```python
from build123d import *

# Parameters (mm, degrees)
SKETCH1_W           = 35
SKETCH1_H           = 22.25
BOSS_EXTRUDE1_DEPTH = 11.5
SKETCH2_R           = 2.2
CUT_EXTRUDE1_DEPTH  = 31.554255023
LPATTERN1_COUNT     = 3
LPATTERN1_PITCH     = 12.7
SKETCH3_W           = 20
SKETCH3_H           = 22.25
BOSS_EXTRUDE2_DEPTH = 50
SKETCH4_W           = 16.4
SKETCH4_H           = 20
BOSS_EXTRUDE3_DEPTH = 44.87
CHAMFER1_SIZE       = 20
SKETCH5_W           = 20
SKETCH5_H           = 22.25
BOSS_EXTRUDE4_DEPTH = 15
CHAMFER2_SIZE       = 12
SKETCH6_W           = 16.4
SKETCH6_H           = 24
BOSS_EXTRUDE5_DEPTH = 18
BOSS_EXTRUDE6_DEPTH = 16.4
SKETCH11_R          = 2.35
CUT_EXTRUDE4_DEPTH  = 119.961327802
SKETCH12_R          = 4.2
CUT_EXTRUDE5_DEPTH  = 16


with BuildPart() as part:
    # Sketch1 → Boss-Extrude1 (new body)
    with BuildSketch(Plane(origin=(0, 0, 0), x_dir=(0, 0, -1), z_dir=(1, 0, 0))):
        Rectangle(SKETCH1_W, SKETCH1_H)
    extrude(amount=BOSS_EXTRUDE1_DEPTH)

    # Sketch2 → Cut-Extrude1 (cut, through all)
    with BuildSketch(Plane(origin=(0, 11.125, 0), x_dir=(1, 0, 0), z_dir=(0, 1, 0))):
        with Locations(Location((5.15, -10.5, 0), (0, 0, 270))):
            Circle(SKETCH2_R)
    cut_extrude1 = extrude(amount=-CUT_EXTRUDE1_DEPTH, mode=Mode.SUBTRACT)

    # LPattern1: Cut-Extrude1 ×3
    with Locations(*[(0, 0, -i * LPATTERN1_PITCH) for i in range(1, LPATTERN1_COUNT)]):
        add(cut_extrude1, mode=Mode.SUBTRACT)


with BuildPart() as body_2:
    # Mirror3: mirrored copy
    add(part.part.mirror(Plane(origin=(43.25, 0, 0), x_dir=(0, 0, 1), z_dir=(1, 0, 0))))


with BuildPart() as part_1:
    add(part.part)

    # Sketch3 → Boss-Extrude2 (add)
    with BuildSketch(Plane(origin=(11.5, 0, 0), x_dir=(0, 0, -1), z_dir=(1, 0, 0))):
        with Locations((7.5, 0)):
            Rectangle(SKETCH3_W, SKETCH3_H)
    extrude(amount=BOSS_EXTRUDE2_DEPTH)

    # Sketch4 → Boss-Extrude3 (add)
    with BuildSketch(Plane(origin=(0, 11.125, 0), x_dir=(1, 0, 0), z_dir=(0, 1, 0))):
        with Locations((53.3, 7.5)):
            Rectangle(SKETCH4_W, SKETCH4_H)
    extrude(amount=BOSS_EXTRUDE3_DEPTH)

    # Chamfer1
    chamfer1_edges = [part_1.edges().sort_by_distance(p)[0] for p in [
        (45.1, 11.125, -7.5),
    ]]
    chamfer(chamfer1_edges, length=CHAMFER1_SIZE)

    add(body_2.part)  # Boss-Extrude4 merges body 2
    # Sketch5 → Boss-Extrude4 (add)
    with BuildSketch(Plane(origin=(61.5, 0, 0), x_dir=(0, 0, -1), z_dir=(1, 0, 0))):
        with Locations((7.5, 0)):
            Rectangle(SKETCH5_W, SKETCH5_H)
    extrude(amount=BOSS_EXTRUDE4_DEPTH)

    # Chamfer2
    chamfer2_edges = [part_1.edges().sort_by_distance(p)[0] for p in [
        (61.5, 11.125, -7.5),
    ]]
    chamfer(chamfer2_edges, length=CHAMFER2_SIZE)

    # Sketch6 → Boss-Extrude5 (add)
    with BuildSketch(Plane(origin=(0, 0, -17.5), x_dir=(-1, 0, 0), z_dir=(0, 0, -1))):
        with Locations((-53.3, 43.995)):
            Rectangle(SKETCH6_W, SKETCH6_H)
    extrude(amount=BOSS_EXTRUDE5_DEPTH)

    # Sketch7 → Boss-Extrude6 (add)
    with BuildSketch(Plane(origin=(61.5, 0, 0), x_dir=(0, 0, -1), z_dir=(1, 0, 0))):
        Polygon((35.5, 31.995), (59.5, 55.995), (35.5, 55.995), align=None)
    extrude(amount=-BOSS_EXTRUDE6_DEPTH)

    # Sketch11 → Cut-Extrude4 (cut, through all)
    with BuildSketch(Plane(origin=(0, -1.7525, -1.7525), x_dir=(1, 0, 0), z_dir=(0, -0.7071067811865509, -0.7071067811865441))):
        with Locations(Location((52.778087488, -58.643931452, 0), (0, 0, 270))):
            Circle(SKETCH11_R)
    extrude(amount=-CUT_EXTRUDE4_DEPTH, mode=Mode.SUBTRACT)

    # Sketch12 → Cut-Extrude5 (cut)
    with BuildSketch(Plane(origin=(0, 17.449710754, 17.449710754), x_dir=(1, 0, 0), z_dir=(0, 0.7071067811865464, 0.7071067811865488))):
        with Locations(Location((52.778087488, 58.643931452, 0), (0, 0, 270))):
            Circle(SKETCH12_R)
    extrude(amount=-CUT_EXTRUDE5_DEPTH, mode=Mode.SUBTRACT)


solid = part_1.part
```
The listing builds one solid part. Answer for the finished solid, in the listing's coordinates (mm). A direction names the side the tool comes from. Give positions to 0.01 mm unless a question says otherwise; leave off trailing zeros. Order: outer loops, then holes, each group sorted by start corner. A loop starts at its lowest first (then second) coordinate and runs counter-clockwise, first axis right, second up. Notation, with made-up numbers: (-35, 22) - (12, 22) arc R19 cw to (12, 43) - close; hole circle Ø11 at (70.25, 73.5). An arc over 180 degrees is marked (long way). Use one line per item in the form item = value. Start each with the question number.
(1) Flat-ended cylindrical pins translate along their axes: pin 1 Ø7.5 at (x, z) = (8, 1) entering from +Y (3 decimals); pin 2 Ø1 at (x, y) = (43.5, 30.5) entering from -Z; pin 3 Ø7.5 at (y, z) = (43.5, -38) entering from -X; pin 4 Ø14.5 at (x, z) = (79.5, 1.5) entering from +Y (3 decimals). Find the tip coordinate at first contact, or state that the pin passes through.
(2) A cutting plane is placed at B-B, the plane x = 81.35. Write down the section's boundary in (y, z) (3 decimals).
(3) A cutting plane is placed at A-A, the plane z = 10.5. Write down the section's boundary in (x, y) (3 decimals), then the cut area to 3 significant figures.
(4) A cutting plane is placed at C-C, the plane z = -14.9. Write down the section's boundary in (x, y) (3 decimals), then the cut area to 3 significant figures.
(5) For faces 1 (the flat face through (53, 31.995, -26)), 2 (the flat face through (61.5, 43, -21)), 3 (the flat face through (11.5, 0, 10)), determine the directions among +Z, -Z, +X, -X, +Y, -Y from which every point of the face is accessible in a straight line to the end or side of a thin tool.
(6) A cutting plane is placed at D-D, the plane x = 18. Write down the section's boundary in (y, z) (3 decimals).
(7) The mould has two halves that part along Y. Classify faces 4 (the cylindrical face through (4.307, 0.156, 12.532)), 5 (the flat face through (12, 11.125, -4)), 6 (the cylindrical face through (55.108, 43.388, -39.115)), 7 (the cylindrical face through (54.04, 49.25, -28.02)): released by +Y, released by -Y, zero draft, split by the parting line, or undercut.
(8) Consider line 1 (Z direction, x = 5, y = 4); line 2 (X direction, y = 0.75, z = 10.5); line 3 (X direction, y = -5.25, z = -14.9). Determine where each line is inside the solid, lowest interval first. Write a range as from..to.
Ans:
q1.pin_1 = 11.125
q1.pin_2 = through
q1.pin_3 = 45.1
q1.pin_4 = 12.375
q2.outline = (-11.125, -17.5) - (11.125, -17.5) - (11.125, -17.1) - (-11.125, -17.1) - close; (-11.125, -12.7) - (11.125, -12.7) - (11.125, -4.4) - (-11.125, -4.4) - close; (-11.125, 0) - (11.125, 0) - (11.125, 8.3) - (-11.125, 8.3) - close; (-11.125, 12.7) - (11.125, 12.7) - (11.125, 17.5) - (-11.125, 17.5) - close
q3.outline = (0, -11.125) - (2.95, -11.125) - (2.95, 11.125) - (0, 11.125) - close; (7.35, -11.125) - (11.5, -11.125) - (11.5, 11.125) - (7.35, 11.125) - close; (75, -11.125) - (79.15, -11.125) - (79.15, 11.125) - (75, 11.125) - close; (83.55, -11.125) - (86.5, -11.125) - (86.5, 11.125) - (83.55, 11.125) - close
q3.area = 316 mm^2
q4.outline = (0, -11.125) - (2.95, -11.125) - (2.95, 11.125) - (0, 11.125) - close; (7.35, -11.125) - (79.15, -11.125) - (79.15, 11.125) - (73.5, 11.125) - (61.5, 23.125) - (61.5, 55.995) - (45.1, 55.995) - (45.1, 31.125) - (25.1, 11.125) - (7.35, 11.125) - close; (83.55, -11.125) - (86.5, -11.125) - (86.5, 11.125) - (83.55, 11.125) - close
q4.area = 2,740 mm^2
q5.face_1 = -Z, +X, -X, -Y
q5.face_2 = +Z, -Z, +X, +Y
q5.face_3 = +Z, +Y, -Y
q6.outline = (-11.125, -17.5) - (11.125, -17.5) - (11.125, 2.5) - (-11.125, 2.5) - close
q7.face_4 = zero draft
q7.face_5 = released by +Y
q7.face_6 = undercut
q7.face_7 = undercut
q8.line_1 = -17.5..-17.09, -12.71..-4.39, -0.01..8.31, 12.69..17.5
q8.line_2 = 0..2.95, 7.35..11.5, 75..79.15, 83.55..86.5
q8.line_3 = 0..2.95, 7.35..79.15, 83.55..86.5
